Build history of the part. All positions in model axes, mm. A direction names the side the tool comes from. Give positions to 0.01 mm unless a question says otherwise; leave off trailing zeros. Loops run counter-clockwise (first coordinate to the right, second up) from the corner with the lowest first, then second, coordinate; pieces in that order, holes last. Notation, with made-up numbers: M 38.5,-23.75 L 50.5,-23.75 A9 ccw 50.5,-16.75 Z; hole C -36,67.25 d1. An arc over 180 degrees is marked long. Answer in a Markdown table with one row per item. Add a question column.
```python
from build123d import *

# Parameters (mm, degrees)
SKETCH1_W           = 38.1
SKETCH1_H           = 156.8323
BOSS_EXTRUDE1_DEPTH = 9.525
FILLET1_R           = 3.048
FILLET2_R           = 3.048
FILLET3_R           = 3.048
SKETCH2_R           = 2.667
CUT_EXTRUDE1_DEPTH  = 25.4
CUT_EXTRUDE2_DEPTH  = 29.718
SKETCH4_R           = 2.667
BOSS_EXTRUDE2_DEPTH = 9.525
SKETCH5_R           = 2.667
CUT_EXTRUDE3_DEPTH  = 9.525


with BuildPart() as part:
    # Sketch1 → Boss-Extrude1 (new body)
    with BuildSketch(Plane(origin=(0, 0, 0), x_dir=(1, 0, 0), z_dir=(0, 1, 0))):
        Rectangle(SKETCH1_W, SKETCH1_H)
    extrude(amount=BOSS_EXTRUDE1_DEPTH)

    # Fillet1
    fillet1_edges = [part.edges().sort_by_distance(p)[0] for p in [
        (19.05, 4.7625, 78.41615),
        (-19.05, 4.7625, 78.41615),
    ]]
    fillet(fillet1_edges, radius=FILLET1_R)

    # Fillet2
    fillet2_edges = [part.edges().sort_by_distance(p)[0] for p in [
        (-19.05, 4.7625, -78.41615),
    ]]
    fillet(fillet2_edges, radius=FILLET2_R)

    # Fillet3
    fillet3_edges = [part.edges().sort_by_distance(p)[0] for p in [
        (19.05, 4.7625, -78.41615),
    ]]
    fillet(fillet3_edges, radius=FILLET3_R)

    # Sketch2 → Cut-Extrude1 (cut)
    with BuildSketch(Plane(origin=(0, 9.525, 0), x_dir=(1, 0, 0), z_dir=(0, 1, 0))):
        with Locations((12.7, 72.06615)):
            Circle(SKETCH2_R)
        with Locations((12.7, -16.83385)):
            Circle(SKETCH2_R)
        with Locations((-12.7, -16.83385)):
            Circle(SKETCH2_R)
        with Locations((-12.7, 72.06615)):
            Circle(SKETCH2_R)
        with Locations((-12.7, -64.25565)):
            Circle(SKETCH2_R)
        with Locations((12.7, -64.25565)):
            Circle(SKETCH2_R)
    extrude(amount=-CUT_EXTRUDE1_DEPTH, mode=Mode.SUBTRACT)

    # Sketch3 → Cut-Extrude2 (cut)
    with BuildSketch(Plane(origin=(0, 9.525, 0), x_dir=(1, 0, 0), z_dir=(0, 1, 0))):
        with BuildLine():
            ThreePointArc((-16.002, -76.95565), (-18.157261469, -76.062911469), (-19.05, -73.90765))
            Line((-19.05, -73.90765), (-19.05, -75.36815))
            ThreePointArc((-19.05, -75.36815), (-18.936369601, -76.19263714), (-18.603950759, -76.95565))
            Line((-18.603950759, -76.95565), (-16.002, -76.95565))
        make_face()
        with BuildLine():
            Line((-12.7, -76.95565), (-16.002, -76.95565))
            Line((-16.002, -76.95565), (-18.603950759, -76.95565))
            ThreePointArc((-18.603950759, -76.95565), (-17.493912196, -78.026063091), (-16.002, -78.41615))
            Line((-16.002, -78.41615), (16.002, -78.41615))
            ThreePointArc((16.002, -78.41615), (17.493912196, -78.026063091), (18.603950759, -76.95565))
            Line((18.603950759, -76.95565), (16.002, -76.95565))
            Line((16.002, -76.95565), (-12.7, -76.95565))
        make_face()
        with BuildLine():
            ThreePointArc((19.05, -73.90765), (18.157261469, -76.062911469), (16.002, -76.95565))
            Line((16.002, -76.95565), (18.603950759, -76.95565))
            ThreePointArc((18.603950759, -76.95565), (18.936369601, -76.19263714), (19.05, -75.36815))
            Line((19.05, -75.36815), (19.05, -73.90765))
        make_face()
    extrude(amount=-CUT_EXTRUDE2_DEPTH, mode=Mode.SUBTRACT)

    # Sketch4 → Boss-Extrude2 (add)
    with BuildSketch(Plane.XZ):
        with BuildLine():
            Line((-92.202, -78.41615), (-16.002, -78.41615))
            ThreePointArc((-16.002, -78.41615), (-18.157261469, -77.523411469), (-19.05, -75.36815))
            Line((-19.05, -75.36815), (-19.05, 26.23185))
            ThreePointArc((-19.05, 26.23185), (-19.942738531, 24.076588531), (-22.098, 23.18385))
            Line((-22.098, 23.18385), (-92.202, 23.18385))
            ThreePointArc((-92.202, 23.18385), (-94.357261469, 22.291111469), (-95.25, 20.13585))
            Line((-95.25, 20.13585), (-95.25, -75.36815))
            ThreePointArc((-95.25, -75.36815), (-94.357261469, -77.523411469), (-92.202, -78.41615))
        make_face()
        with Locations((-88.9, -72.06615)):
            Circle(SKETCH4_R, mode=Mode.SUBTRACT)
        with Locations((-63.5, -72.06615)):
            Circle(SKETCH4_R, mode=Mode.SUBTRACT)
        with Locations((-38.1, -72.06615)):
            Circle(SKETCH4_R, mode=Mode.SUBTRACT)
        with Locations((-88.9, 16.83385)):
            Circle(SKETCH4_R, mode=Mode.SUBTRACT)
        with Locations((-63.5, 16.83385)):
            Circle(SKETCH4_R, mode=Mode.SUBTRACT)
        with Locations((-38.1, 16.83385)):
            Circle(SKETCH4_R, mode=Mode.SUBTRACT)
    extrude(amount=-BOSS_EXTRUDE2_DEPTH)

    # Sketch5 → Cut-Extrude3 (cut)
    with BuildSketch(Plane.XZ):
        with Locations((0, -21.26615)):
            Circle(SKETCH5_R)
        with Locations((-76.2, -21.26615)):
            Circle(SKETCH5_R)
    extrude(amount=-CUT_EXTRUDE3_DEPTH, mode=Mode.SUBTRACT)


solid = part.part
```
(1) Slice it at C-C, the plane x = 0. Give the cut face in (y, z) (3 decimals), then the cut area to 3 significant figures.
(2) Pull direction Z, two halves, no side cores. Call faces 3 (the flat face through (-39, 5, -78.416)), 4 (the cylindrical face through (-19.92, 4.7, 24.1)), 5 (the cylindrical face through (-62.066, 4.696, -69.817)): +Z half, -Z half, draft (parallel to the pull), parting line (faces both ways), or undercut.
(3) Slice it at D-D, the plane y = 8. State how many separate pieces and enclosed holes the cut face has, then the cut area to 3 significant figures.
(4) Slice it at B-B, the plane x = 12.7. Give the cut face in (y, z) (3 decimals).
(5) Pin check, flat tip, straight feed: pin 1 (5 mm diameter, centred on y = 4, z = 54, fed in from -X). Stop position of the tip, or through.
(6) Wall check: line 1 (Z direction, x = -63.5, y = 3.5); line 2 (Z direction, x = 0, y = 6.25); line 3 (Z direction, x = -66.5, y = 1.5). Give the ranges that are in metal, low to high.
(7) Tool access for faces 1 (the flat face through (-57, 5, 23.184)), 2 (the cylindrical face through (-38.447, 4.696, -69.422)): list every direction of +Z, -Z, +X, -X, +Y, -Y with a clear straight run to the whole face (end or side of a thin tool).
(8) Slice it at A-A, the plane x = -38.1. Give the cut face in (y, z) (3 decimals), then the cut area to 3 significant figures.
Solution:
| question | item | result |
|---|---|---|
| 1 | outline | M 0,-78.416 L 9.525,-78.416 L 9.525,-23.933 L 0,-23.933 Z; M 0,-18.599 L 9.525,-18.599 L 9.525,76.956 L 0,76.956 Z |
| 1 | area | 1,430 mm^2 |
| 2 | face 3 | -Z half |
| 2 | face 4 | +Z half |
| 2 | face 5 | undercut |
| 3 | separate pieces | 1 |
| 3 | enclosed holes | 14 |
| 3 | area | 13,300 mm^2 |
| 4 | outline | M 0,-78.416 L 9.525,-78.416 L 9.525,-74.733 L 0,-74.733 Z; M 0,-69.399 L 9.525,-69.399 L 9.525,14.167 L 0,14.167 Z; M 0,19.501 L 9.525,19.501 L 9.525,61.589 L 0,61.589 Z; M 0,66.923 L 9.525,66.923 L 9.525,76.956 L 0,76.956 Z |
| 5 | pin 1 | x = -19.05 |
| 6 | line 1 | -78.42 to -74.73, -69.4 to 14.17, 19.5 to 23.18 |
| 6 | line 2 | -78.42 to -23.93, -18.6 to 76.96 |
| 6 | line 3 | -78.42 to 23.18 |
| 7 | face 1 | +Z, -X, +Y, -Y |
| 7 | face 2 | +Y, -Y |
| 8 | outline | M 0,-78.416 L 9.525,-78.416 L 9.525,-74.733 L 0,-74.733 Z; M 0,-69.399 L 9.525,-69.399 L 9.525,14.167 L 0,14.167 Z; M 0,19.501 L 9.525,19.501 L 9.525,23.184 L 0,23.184 Z |
| 8 | area | 866 mm^2 |
